```python
from build123d import *

# Parameters (mm, degrees)
SKETCH1_W           = 69.85
SKETCH1_H           = 38.1
BOSS_EXTRUDE1_DEPTH = 2.84
SKETCH2_W           = 11.1125
SKETCH2_H           = 10.23
BOSS_EXTRUDE5_DEPTH = 20
SKETCH4_W           = 3.192184281
SKETCH4_H           = 38.1
BOSS_EXTRUDE7_DEPTH = 38.1
FILLET1_R           = 5.55625
FILLET2_R           = 5.55625
SKETCH5_W           = 8
SKETCH5_H           = 14.5
CUT_EXTRUDE1_DEPTH  = 38.1
SKETCH6_W           = 5.25
SKETCH6_H           = 5.25
CUT_EXTRUDE2_DEPTH  = 10
SKETCH7_W           = 5.253
SKETCH7_H           = 5.25
CUT_EXTRUDE3_DEPTH  = 10
SKETCH8_R           = 2.38125
CUT_EXTRUDE4_DEPTH  = 10
SKETCH9_R           = 2.38125
CUT_EXTRUDE5_DEPTH  = 10
SKETCH10_W          = 4.5
SKETCH10_H          = 14.5
CUT_EXTRUDE6_DEPTH  = 10
SKETCH12_R          = 2.38125
CUT_EXTRUDE7_DEPTH  = 10
SKETCH13_R          = 2.38125
CUT_EXTRUDE8_DEPTH  = 10


with BuildPart() as part:
    # Sketch1 → Boss-Extrude1 (new body)
    with BuildSketch(Plane(origin=(0, 0, 0), x_dir=(1, 0, 0), z_dir=(0, 1, 0))):
        with Locations((-22.809987281, -11.136378688)):
            Rectangle(SKETCH1_W, SKETCH1_H)
    extrude(amount=BOSS_EXTRUDE1_DEPTH)

    # Sketch2 → Boss-Extrude5 (add)
    with BuildSketch(Plane(origin=(0, 2.84, 0), x_dir=(1, 0, 0), z_dir=(0, 1, 0))):
        with Locations((-21.968737281, -11.491378688)):
            Rectangle(SKETCH2_W, SKETCH2_H)
    extrude(amount=BOSS_EXTRUDE5_DEPTH)

    # Sketch4 → Boss-Extrude7 (add)
    with BuildSketch(Plane(origin=(0, 2.84, 0), x_dir=(1, 0, 0), z_dir=(0, 1, 0))):
        with Locations((-30.721079422, -11.136378688)):
            Rectangle(SKETCH4_W, SKETCH4_H)
    extrude(amount=BOSS_EXTRUDE7_DEPTH)

    # Fillet1
    fillet1_edges = [part.edges().sort_by_distance(p)[0] for p in [
        (-16.412487281, 22.84, 11.491378688),
    ]]
    fillet(fillet1_edges, radius=FILLET1_R)

    # Fillet2
    fillet2_edges = [part.edges().sort_by_distance(p)[0] for p in [
        (-27.524987281, 22.84, 11.491378688),
    ]]
    fillet(fillet2_edges, radius=FILLET2_R - 0.0001)  # a hair under: the kernel refuses the full size

    # Sketch5 → Cut-Extrude1 (cut)
    with BuildSketch(Plane(origin=(0, 2.84, 0), x_dir=(1, 0, 0), z_dir=(0, 1, 0))):
        with Locations((-40.817171562, -10.386378688)):
            Rectangle(SKETCH5_W, SKETCH5_H)
    extrude(amount=-CUT_EXTRUDE1_DEPTH, mode=Mode.SUBTRACT)

    # Sketch6 → Cut-Extrude2 (cut)
    with BuildSketch(Plane(origin=(-29.124987281, 0, 0), x_dir=(0, 0, -1), z_dir=(1, 0, 0))):
        with Locations((2.538621312, 7.965)):
            Rectangle(SKETCH6_W, SKETCH6_H)
    extrude(amount=-CUT_EXTRUDE2_DEPTH, mode=Mode.SUBTRACT)

    # Sketch7 → Cut-Extrude3 (cut)
    with BuildSketch(Plane(origin=(-29.124987281, 0, 0), x_dir=(0, 0, -1), z_dir=(1, 0, 0))):
        with Locations((-24.809878688, 7.965)):
            Rectangle(SKETCH7_W, SKETCH7_H)
    extrude(amount=-CUT_EXTRUDE3_DEPTH, mode=Mode.SUBTRACT)

    # Sketch8 → Cut-Extrude4 (cut)
    with BuildSketch(Plane(origin=(0, 2.84, 0), x_dir=(1, 0, 0), z_dir=(0, 1, 0))):
        with Locations(Location((8.415012719, 4.213621312, 0), (0, 0, 270))):
            Circle(SKETCH8_R)
    extrude(amount=-CUT_EXTRUDE4_DEPTH, mode=Mode.SUBTRACT)

    # Sketch9 → Cut-Extrude5 (cut)
    with BuildSketch(Plane(origin=(0, 2.84, 0), x_dir=(1, 0, 0), z_dir=(0, 1, 0))):
        with Locations(Location((8.415012719, -26.486378688, 0), (0, 0, 270))):
            Circle(SKETCH9_R)
    extrude(amount=-CUT_EXTRUDE5_DEPTH, mode=Mode.SUBTRACT)

    # Sketch10 → Cut-Extrude6 (cut)
    with BuildSketch(Plane(origin=(0, 2.84, 0), x_dir=(1, 0, 0), z_dir=(0, 1, 0))):
        with Locations((-34.567171562, -10.386378688)):
            Rectangle(SKETCH10_W, SKETCH10_H)
    extrude(amount=-CUT_EXTRUDE6_DEPTH, mode=Mode.SUBTRACT)

    # Sketch12 → Cut-Extrude7 (cut)
    with BuildSketch(Plane(origin=(0, 2.84, 0), x_dir=(1, 0, 0), z_dir=(0, 1, 0))):
        with Locations(Location((-54.034987281, -26.486378688, 0), (0, 0, 270))):
            Circle(SKETCH12_R)
    extrude(amount=-CUT_EXTRUDE7_DEPTH, mode=Mode.SUBTRACT)

    # Sketch13 → Cut-Extrude8 (cut)
    with BuildSketch(Plane(origin=(0, 2.84, 0), x_dir=(1, 0, 0), z_dir=(0, 1, 0))):
        with Locations(Location((-54.034987281, 4.213621312, 0), (0, 0, 270))):
            Circle(SKETCH13_R)
    extrude(amount=-CUT_EXTRUDE8_DEPTH, mode=Mode.SUBTRACT)


solid = part.part
```
CAD build for the part. Positions are in the model's coordinates, mm. A direction names the side the tool comes from. Round coordinates to 2 decimals unless told otherwise and drop trailing zeros. Loops run counter-clockwise (first coordinate to the right, second up) from the corner with the lowest first, then second, coordinate; pieces in that order, holes last. Notation, with made-up numbers: M 43.25,-20 L 99.25,-20 A10 ccw 99.25,-9 Z; hole C 16.5,58.5 d8. An arc over 180 degrees is marked long. Return JSON: item names as keys, results as strings. Group by question number.
(1) Saw through at D-D, the plane z = 18.5. List the corners of the cut face in (x, y), and give its area (3 significant figures).
(2) Wall check: probe 1 along X at (y, z) = (14, 15); probe 2 along Y at (x, z) = (-17, -1); probe 3 along X at (y, z) = (14.5, 20.5). Give the ranges that are in metal, low to high. Write a range as [from, to].
(3) Tool access for faces 4 (the flat face through (-45, 2.84, 11)), 5 (the flat face through (-31, 8, 27.436)), 6 (the flat face through (-16.412, 10, 12)), 7 (the flat face through (-39, 1, 3.136)): list every direction of +Z, -Z, +X, -X, +Y, -Y with a clear straight run to the whole face (end or side of a thin tool).
(4) Saw through at C-C, the plane y = 14. List the corners of the cut face in (x, z).
(5) Mould opens along Z. For faces 1 (the flat face through (-22, 13, 6.376)), 2 (the flat face through (-31, 40.94, 11)), 3 (the cylindrical face through (-56.36, 1.44, -4.73)) say: +Z half, -Z half, draft (parallel to the pull), parting line (faces both ways), or undercut.
(6) Saw through at A-A, the plane z = 23. List the corners of the cut face in (x, y).
(7) Saw through at B-B, the plane x = -37. List the corners of the cut face in (y, z).
(8) Drop flat-ended pins along their axis: P1, Ø1.6, axis at x = -30.5, z = -2, coming from the -Y side; P2, Ø11.5, axis at y = 28, z = 14.5, coming from the -X side; P3, Ø8, axis at y = 21.5, z = -0.5, coming from the +X side (3 decimals); P4, Ø10, axis at x = -49, z = 23, coming from the +Y side. Give the stop position or say it passes through.
Answer list:
{
 "1": {"outline": "M -57.73,0 L 12.12,0 L 12.12,2.84 L -29.12,2.84 L -29.12,40.94 L -32.32,40.94 L -32.32,2.84 L -57.73,2.84 Z", "area": "320 mm2"},
 "2": {"probe 1": "[-32.32, -29.12], [-27.52, -16.41]", "probe 2": "[0, 2.84]", "probe 3": "[-32.32, -29.12]"},
 "3": {"face 4": "+Z, -Z, -X, +Y", "face 5": "+X, -X", "face 6": "+Z, -Z, +X, +Y", "face 7": "+Y, -Y"},
 "4": {"outline": "M -32.32,-7.91 L -29.12,-7.91 L -29.12,30.19 L -32.32,30.19 Z; M -27.52,6.38 L -16.41,6.38 L -16.41,16.61 L -27.52,16.61 Z"},
 "5": {"face 1": "-Z half", "face 2": "draft", "face 3": "undercut"},
 "6": {"outline": "M -57.73,0 L 12.12,0 L 12.12,2.84 L -29.12,2.84 L -29.12,5.34 L -32.32,5.34 L -32.32,2.84 L -57.73,2.84 Z; M -32.32,10.59 L -29.12,10.59 L -29.12,40.94 L -32.32,40.94 Z"},
 "7": {"outline": "M 0,-7.91 L 2.84,-7.91 L 2.84,3.14 L 0,3.14 Z; M 0,17.64 L 2.84,17.64 L 2.84,30.19 L 0,30.19 Z"},
 "8": {"P1": "y = 0", "P2": "x = -32.32", "P3": "x = -29.125", "P4": "y = 2.84"}
}
